Check sheet for the modelled part. Datum: model origin and axes. Units: mm. A direction names the side the tool comes from. Round coordinates to 2 decimals unless told otherwise and drop trailing zeros. Loops run counter-clockwise (first coordinate to the right, second up) from the corner with the lowest first, then second, coordinate; pieces in that order, holes last. Notation, with made-up numbers: (74, 83) - (98, 83) arc R16 ccw to (98, 105) - close; hole circle Ø11 at (-35.75, 84). An arc over 180 degrees is marked (long way). Put each result on its own line as item: value. Start each with the question number.
```python
from build123d import *

# Parameters (mm, degrees)
BOSS_EXTRUDE1_DEPTH = 2
BOSS_EXTRUDE2_START = 4.5
BOSS_EXTRUDE2_DEPTH = 4.5
CUT_EXTRUDE1_DEPTH  = 4.5
BOSS_EXTRUDE3_DEPTH = 2.3
SKETCH9_R           = 2.1
CUT_EXTRUDE2_DEPTH  = 2.5
SKETCH10_R          = 2.5
BOSS_EXTRUDE4_DEPTH = 1.2
SKETCH11_R          = 0.95
CUT_EXTRUDE3_DEPTH  = 9.2
SKETCH12_R          = 2
CUT_EXTRUDE4_DEPTH  = 4.5
SKETCH14_W          = 20.343145751
SKETCH14_H          = 1.841510486
SKETCH14_W_2        = 17
SKETCH14_H_2        = 1.341637015
BOSS_EXTRUDE5_DEPTH = 1.2
FILLET1_R           = 1.5
SKETCH17_R          = 0.95
CUT_EXTRUDE5_DEPTH  = 3


# Read off the part's stored shape, not the designer's step: Boss-Extrude3
with BuildPart() as part:
    # Sketch5 → Boss-Extrude1 (new body)
    with BuildSketch(Plane.XY):
        with BuildLine():
            Line((8, 0), (9, -2.501635265))
            Line((9, -2.501635265), (9, -7.001635265))
            Line((9, -7.001635265), (26, -7.001635265))
            Line((26, -7.001635265), (26, 7.498364735))
            Line((26, 7.498364735), (5.656854249, 7.498364735))
            Line((5.656854249, 7.498364735), (5.656854249, 5.656854249))
            ThreePointArc((5.656854249, 5.656854249), (7.39103626, 3.061467459), (8, 0))
        make_face()
    extrude(amount=BOSS_EXTRUDE1_DEPTH)

    # Sketch6 → Boss-Extrude2 (add)
    with BuildSketch(Plane(origin=(0, 0, 0), x_dir=(-1, 0, 0), z_dir=(0, 0, -1)).offset(BOSS_EXTRUDE2_START)):
        with BuildLine():
            Line((-5.656854249, 7.498364735), (-5.656854249, 5.656854249))
            ThreePointArc((-5.656854249, 5.656854249), (-7.39103626, 3.061467459), (-8, 0))
            Line((-8, 0), (-9, -2.501635265))
            Line((-9, -2.501635265), (-9, -7.001635265))
            Line((-9, -7.001635265), (-26, -7.001635265))
            Line((-26, -7.001635265), (-26, 7.498364735))
            Line((-26, 7.498364735), (-5.656854249, 7.498364735))
        make_face()
    extrude(amount=-BOSS_EXTRUDE2_DEPTH)

    # Sketch7 → Cut-Extrude1 (cut)
    with BuildSketch(Plane(origin=(0, 0, -4.5), x_dir=(-1, 0, 0), z_dir=(0, 0, -1))):
        Polygon((-26, 5.298364735), (-2.738141148, 5.298364735), (-2.738141148, 3.998364735), (-29.849535112, 3.998364735), (-29.849535112, 5.298364735), align=None)
    extrude(amount=-CUT_EXTRUDE1_DEPTH, mode=Mode.SUBTRACT)

    # Boss-Extrude3 outline → Boss-Extrude3 (add)
    with BuildSketch(Plane(origin=(0, 0, -4.5), x_dir=(-1, 0, 0), z_dir=(0, 0, -1))):
        with BuildLine():
            Line((-9, -7.001635265), (-9, -5.65999825))
            Line((-9, -5.65999825), (0, -5.659997813))
            ThreePointArc((0, -5.659997813), (5.659997813, 0), (0, 5.659997813))
            Line((0, 5.659997813), (-5.656854249, 5.656854249))
            Line((-5.656854249, 5.656854249), (-5.656854249, 7.498364735))
            Line((-5.656854249, 7.498364735), (-26, 7.498364735))
            Line((-26, 7.498364735), (-26, -7.001635265))
            Line((-26, -7.001635265), (-9, -7.001635265))
        make_face()
    extrude(amount=BOSS_EXTRUDE3_DEPTH)

    # Sketch9 → Cut-Extrude2 (cut)
    with BuildSketch(Plane(origin=(0, 0, -6.8), x_dir=(-1, 0, 0), z_dir=(0, 0, -1))):
        Circle(SKETCH9_R)
    extrude(amount=-CUT_EXTRUDE2_DEPTH, mode=Mode.SUBTRACT)

    # Sketch10 → Boss-Extrude4 (add)
    with BuildSketch(Plane(origin=(0, 0, -6.8), x_dir=(-1, 0, 0), z_dir=(0, 0, -1))):
        with Locations((-12, 0)):
            Circle(SKETCH10_R)
        with Locations((-18, 0)):
            Circle(SKETCH10_R)
    extrude(amount=BOSS_EXTRUDE4_DEPTH)

    # Sketch11 → Cut-Extrude3 (cut)
    with BuildSketch(Plane(origin=(0, 0, -8), x_dir=(-1, 0, 0), z_dir=(0, 0, -1))):
        with Locations((-18, 0)):
            Circle(SKETCH11_R)
        with Locations((-12, 0)):
            Circle(SKETCH11_R)
    extrude(amount=-CUT_EXTRUDE3_DEPTH, mode=Mode.SUBTRACT)

    # Sketch12 → Cut-Extrude4 (cut)
    with BuildSketch(Plane.XY.offset(2)):
        with Locations((12, 0)):
            Circle(SKETCH12_R)
        with Locations((18, 0)):
            Circle(SKETCH12_R)
    extrude(amount=-CUT_EXTRUDE4_DEPTH, mode=Mode.SUBTRACT)

    # Sketch14 → Boss-Extrude5 (add)
    with BuildSketch(Plane(origin=(0, 0, -6.8), x_dir=(-1, 0, 0), z_dir=(0, 0, -1))):
        with Locations((-15.828427124, 6.577609492)):
            Rectangle(SKETCH14_W, SKETCH14_H)
        with Locations((-17.5, -6.330816758)):
            Rectangle(SKETCH14_W_2, SKETCH14_H_2)
    extrude(amount=BOSS_EXTRUDE5_DEPTH)

    # Fillet1
    # the kernel refuses this fillet: 1.5 mm, written as the material it takes off along each edge
    with BuildSketch(Plane(origin=(24.5, -5.501635265, 0.5), x_dir=(0, 0, 1), z_dir=(0, -1, 0))) as fillet1_piece_1_section:
        Polygon((0, 0), (FILLET1_R, 0), (FILLET1_R, -FILLET1_R), (0, -FILLET1_R), align=None)
    fillet1_piece_1 = extrude(amount=FILLET1_R, mode=Mode.PRIVATE)
    fillet1_piece_1 = fillet1_piece_1 - Plane(origin=(24.5, -5.501635265, 0.5), x_dir=(-0.7071067811865475, 0, -0.7071067811865475), z_dir=(0, -1, 0)) * Sphere(FILLET1_R, mode=Mode.PRIVATE)
    add(fillet1_piece_1, mode=Mode.SUBTRACT)
    with BuildSketch(Plane(origin=(24.5, 5.998364735, 0.5), x_dir=(0, 0, 1), z_dir=(0, 1, 0))) as fillet1_piece_2_section:
        Polygon((0, 0), (FILLET1_R, 0), (FILLET1_R, FILLET1_R), (0, FILLET1_R), align=None)
    fillet1_piece_2 = extrude(amount=FILLET1_R, mode=Mode.PRIVATE)
    fillet1_piece_2 = fillet1_piece_2 - Plane(origin=(24.5, 5.998364735, 0.5), x_dir=(-0.7071067811865475, 0, -0.7071067811865475), z_dir=(0, 1, 0)) * Sphere(FILLET1_R, mode=Mode.PRIVATE)
    add(fillet1_piece_2, mode=Mode.SUBTRACT)
    with BuildSketch(Plane(origin=(26, -5.501635265, 2), x_dir=(-1, 0, 0), z_dir=(0, 1, 0))) as fillet1_piece_3:
        with BuildLine():
            CenterArc((FILLET1_R, -FILLET1_R), FILLET1_R, 90, 90)
            Line((0, -FILLET1_R), (0, 0))
            Line((0, 0), (FILLET1_R, 0))
        make_face()
    extrude(amount=11.5, mode=Mode.SUBTRACT)
    with BuildSketch(Plane(origin=(26, -7.001635265, -4.5), x_dir=(-1, 0, 0), z_dir=(0, 0, 1))) as fillet1_piece_4:
        with BuildLine():
            CenterArc((FILLET1_R, -FILLET1_R), FILLET1_R, 90, 90)
            Line((0, -FILLET1_R), (0, 0))
            Line((0, 0), (FILLET1_R, 0))
        make_face()
    extrude(amount=5, mode=Mode.SUBTRACT)
    with BuildSketch(Plane(origin=(5.25, -7.001635265, 2), x_dir=(0, 1, 0), z_dir=(1, 0, 0))) as fillet1_piece_5:
        with BuildLine():
            CenterArc((FILLET1_R, -FILLET1_R), FILLET1_R, 90, 90)
            Line((0, -FILLET1_R), (0, 0))
            Line((0, 0), (FILLET1_R, 0))
        make_face()
    extrude(amount=19.25, mode=Mode.SUBTRACT)
    with BuildSketch(Plane(origin=(24.5, 7.498364735, 2), x_dir=(0, -1, 0), z_dir=(-1, 0, 0))) as fillet1_piece_6:
        with BuildLine():
            CenterArc((FILLET1_R, -FILLET1_R), FILLET1_R, 90, 90)
            Line((0, -FILLET1_R), (0, 0))
            Line((0, 0), (FILLET1_R, 0))
        make_face()
    extrude(amount=22.593145751, mode=Mode.SUBTRACT)
    with BuildSketch(Plane(origin=(26, 7.498364735, -4.5), x_dir=(-1, 0, 0), z_dir=(0, 0, 1))) as fillet1_piece_7:
        with BuildLine():
            CenterArc((FILLET1_R, FILLET1_R), FILLET1_R, 180, 90)
            Line((0, FILLET1_R), (0, 0))
            Line((0, 0), (FILLET1_R, 0))
        make_face()
    extrude(amount=5, mode=Mode.SUBTRACT)
    with BuildSketch(Plane(origin=(26, 7.498364735, -4.5), x_dir=(-1.0, -1.9174232572065026e-10, 0), z_dir=(0, 0, -1))) as fillet1_piece_8:
        with BuildLine():
            CenterArc((FILLET1_R, -FILLET1_R), FILLET1_R, 90.000000011, 90)
            Line((FILLET1_R * 1.9173522033e-10, -FILLET1_R), (0, 0))
            Line((0, 0), (FILLET1_R, 0))
        make_face()
    extrude(amount=2.3, mode=Mode.SUBTRACT)
    with BuildSketch(Plane(origin=(26, 7.498364735, -6.8), x_dir=(-1, 0, 0), z_dir=(0, 0, -1))) as fillet1_piece_9:
        with BuildLine():
            CenterArc((FILLET1_R, -FILLET1_R), FILLET1_R, 90, 90)
            Line((0, -FILLET1_R), (0, 0))
            Line((0, 0), (FILLET1_R, 0))
        make_face()
    extrude(amount=4.95, mode=Mode.SUBTRACT)
    with BuildSketch(Plane(origin=(26, -7.001635265, -4.5), x_dir=(-1.0, -1.9169850891861218e-10, 0), z_dir=(0, 0, -1))) as fillet1_piece_10:
        with BuildLine():
            CenterArc((FILLET1_R, FILLET1_R), FILLET1_R, 180.000000011, 90)
            Line((-FILLET1_R * 1.91707982785e-10, FILLET1_R), (0, 0))
            Line((0, 0), (FILLET1_R, 0))
        make_face()
    extrude(amount=2.3, mode=Mode.SUBTRACT)
    with BuildSketch(Plane(origin=(26, -7.001635265, -6.8), x_dir=(-1, 0, 0), z_dir=(0, 0, -1))) as fillet1_piece_11:
        with BuildLine():
            CenterArc((FILLET1_R, FILLET1_R), FILLET1_R, 180, 90)
            Line((0, FILLET1_R), (0, 0))
            Line((0, 0), (FILLET1_R, 0))
        make_face()
    extrude(amount=4.95, mode=Mode.SUBTRACT)

    # Sketch17 → Cut-Extrude5 (cut)
    with BuildSketch(Plane.XZ.offset(7.001635265)):
        with Locations((22, -1)):
            Circle(SKETCH17_R)
        with Locations((18, -1)):
            Circle(SKETCH17_R)
    extrude(amount=-CUT_EXTRUDE5_DEPTH, mode=Mode.SUBTRACT)

    # Mirror1: part across plane


with BuildPart() as part_1:
    add(part.part)
    add(part.part.mirror(Plane(origin=(0, 0, -8), x_dir=(1, 0, 0), z_dir=(0, 0, -1))))


with BuildPart() as body_2:
    # Split1: the piece on the far side of the plane
    add(part_1.part)
    split(bisect_by=Plane(origin=(0, 0, -8), x_dir=(-1, 0, 0), z_dir=(0, 0, -1)), keep=Keep.BOTTOM)


with BuildPart() as part_2:
    add(part_1.part)

    # Split1
    split(bisect_by=Plane(origin=(0, 0, -8), x_dir=(-1, 0, 0), z_dir=(0, 0, -1)), keep=Keep.TOP)


with BuildPart() as body_2_2:
    # Split2: the piece on the far side of the plane
    add(part_2.part)
    split(bisect_by=Plane(origin=(0, 0, -11.5), x_dir=(-1, 0, 0), z_dir=(0, 0, -1)), keep=Keep.BOTTOM)


with BuildPart() as part_3:
    add(part_2.part)

    # Split2
    split(bisect_by=Plane(origin=(0, 0, -11.5), x_dir=(-1, 0, 0), z_dir=(0, 0, -1)), keep=Keep.TOP)


solid = part_3.part
```
Q1. Material ranges on line 1 (Y direction, x = 12, z = -13.1); line 2 (Y direction, x = 12, z = -15); line 3 (X direction, y = -5.4, z = -15), recorded low to high. Write a range as from..to.
Q2. Cross-section at A-A on z = -13.25. Enter the section's corners in (x, y), and give its area (3 significant figures).
Q3. Depth check by flat-ended pin: pin 1 Ø1.2 at (x, y) = (18, -0.5) entering from -Z; pin 2 Ø1.7 at (x, y) = (18, 0) entering from -Z; pin 3 Ø6.5 at (x, y) = (18, 0) entering from +Z; pin 4 Ø0.9 at (x, z) = (18, -15) entering from -Y. Enter the tip coordinate at first touch or a pass-through.
Q4. Draft check along Y on faces 1 (the face through (17, -7.002, -14)), 2 (the face through (16, 5.298, -14)), 3 (the face through (5.657, 7, -15)). Enter one of: +Y half, -Y half, draft (parallel to the pull), parting line (faces both ways), or undercut.
Q5. Cross-section at D-D on x = 22. Enter the section's corners in (y, z).
Q6. Set-up check for faces 4 (the face through (22, -4.002, -15)), 5 (the face through (10.4, -1.2, -15.8)), 6 (the face through (9, -5, -15)): record each of +Z, -Z, +X, -X, +Y, -Y from which the full face is reachable in a straight line by a thin tool's end or side.
Q7. Cross-section at B-B on x = 18. Enter the section's corners in (y, z), and give its area (3 significant figures).
Q8. Cross-section at C-C on z = -15. Enter the section's corners in (x, y).
Answer list:
1. line 1: y = -7..-0.95, 0.95..4, 5.3..7.5
1. line 2: y = -7..-2, 2..4, 5.3..7.5
1. line 3: x = 9..17.05, 18.95..21.05, 22.95..26
2. outline: (5.66, 5.66) arc R8 cw to (5.99, 5.3) - (26, 5.3) - (26, 6) arc R1.5 ccw to (24.5, 7.5) - (5.66, 7.5) - close; (6.93, 4) arc R8 cw to (8, 0) - (9, -2.5) - (9, -7) - (24.5, -7) arc R1.5 ccw to (26, -5.5) - (26, 4) - close; hole circle Ø1.9 at (12, 0); hole circle Ø1.9 at (18, 0)
2. area: 232 mm2
3. pin 1: stops at z = -13.5
3. pin 2: passes through
3. pin 3: stops at z = -11.5
3. pin 4: stops at y = -4
4. face 1: -Y half
4. face 2: undercut
4. face 3: draft
5. outline: (-7, -16.5) arc R1.5 ccw to (-5.5, -18) - (6, -18) arc R1.5 ccw to (7.5, -16.5) - (7.5, -11.5) - (5.3, -11.5) - (5.3, -16) - (4, -16) - (4, -11.5) - (-7, -11.5) - (-7, -14.05) - (-4, -14.05) - (-4, -15.95) - (-7, -15.95) - close
6. face 4: -Y
6. face 5: -Z
6. face 6: +Z, -Z, -X, -Y
7. outline: (-7, -16.5) arc R1.5 ccw to (-5.5, -18) - (-2, -18) - (-2, -13.5) - (-0.95, -13.5) - (-0.95, -11.5) - (-7, -11.5) - (-7, -14.05) - (-4, -14.05) - (-4, -15.95) - (-7, -15.95) - close; (0.95, -13.5) - (2, -13.5) - (2, -18) - (6, -18) arc R1.5 ccw to (7.5, -16.5) - (7.5, -11.5) - (5.3, -11.5) - (5.3, -16) - (4, -16) - (4, -11.5) - (0.95, -11.5) - close
7. area: 59.9 mm2
8. outline: (5.66, 5.66) arc R8 cw to (5.99, 5.3) - (26, 5.3) - (26, 6) arc R1.5 ccw to (24.5, 7.5) - (5.66, 7.5) - close; (6.93, 4) arc R8 cw to (8, 0) - (9, -2.5) - (9, -7) - (17.05, -7) - (17.05, -4) - (18.95, -4) - (18.95, -7) - (21.05, -7) - (21.05, -4) - (22.95, -4) - (22.95, -7) - (24.5, -7) arc R1.5 ccw to (26, -5.5) - (26, 4) - close; hole circle Ø4 at (12, 0); hole circle Ø4 at (18, 0)
